```python
from build123d import *

# Parameters (mm, degrees)
SKETCH_1_R      = 6
SKETCH_1_R_2    = 5.25
EXTRUDE_2_DEPTH = 40
SKETCH_2_R      = 7.5
EXTRUDE_3_DEPTH = 3
SKETCH_3_R      = 5
EXTRUDE_4_DEPTH = 190
EXTRUDE_6_DEPTH = 1.8


with BuildPart() as part:
    # 草图1 → 凸台-拉伸2 (new body)
    with BuildSketch(Plane(origin=(0, 0, 0), x_dir=(1, 0, 0), z_dir=(0, 1, 0))):
        with Locations(Location((0, 0, 0), (0, 0, 270))):
            Circle(SKETCH_1_R)
        with Locations(Location((0, 0, 0), (0, 0, 270))):
            Circle(SKETCH_1_R_2, mode=Mode.SUBTRACT)
    extrude(amount=EXTRUDE_2_DEPTH)

    # 草图2 → 凸台-拉伸3 (add)
    with BuildSketch(Plane(origin=(0, 40, 0), x_dir=(1, 0, 0), z_dir=(0, 1, 0))):
        with Locations(Location((0, 0, 0), (0, 0, 270))):
            Circle(SKETCH_2_R)
    extrude(amount=EXTRUDE_3_DEPTH)

    # 草图3 → 凸台-拉伸4 (add)
    with BuildSketch(Plane(origin=(0, 43, 0), x_dir=(1, 0, 0), z_dir=(0, 1, 0))):
        with Locations(Location((0, 0, 0), (0, 0, 270))):
            Circle(SKETCH_3_R)
    extrude(amount=EXTRUDE_4_DEPTH)

    # 草图4 → 凸台-拉伸6 (add)
    with BuildSketch(Plane(origin=(0, 43, 0), x_dir=(1, 0, 0), z_dir=(0, 1, 0))):
        with BuildLine():
            Line((6, 2.2), (4.489988864, 2.2))
            ThreePointArc((4.489988864, 2.2), (4.870828693, 1.129171307), (5, 0))
            ThreePointArc((5, 0), (4.870828693, -1.129171307), (4.489988864, -2.2))
            Line((4.489988864, -2.2), (6, -2.2))
            Line((6, -2.2), (6, 2.2))
        make_face()
        with BuildLine():
            ThreePointArc((2.2, -4.489988864), (0, -5), (-2.2, -4.489988864))
            Line((-2.2, -4.489988864), (-2.2, -6))
            Line((-2.2, -6), (2.2, -6))
            Line((2.2, -6), (2.2, -4.489988864))
        make_face()
        with BuildLine():
            Line((-2.2, 6), (-2.2, 4.489988864))
            ThreePointArc((-2.2, 4.489988864), (0, 5), (2.2, 4.489988864))
            Line((2.2, 4.489988864), (2.2, 6))
            Line((2.2, 6), (-2.2, 6))
        make_face()
        with BuildLine():
            ThreePointArc((-4.489988864, -2.2), (-5, 0), (-4.489988864, 2.2))
            Line((-4.489988864, 2.2), (-6, 2.2))
            Line((-6, 2.2), (-6, -2.2))
            Line((-6, -2.2), (-4.489988864, -2.2))
        make_face()
    extrude(amount=EXTRUDE_6_DEPTH)


solid = part.part
```
Here's how the part is built. I have some questions about the finished solid (model axes, mm). A direction names the side the tool comes from. Coordinates: 2 decimals unless noted, no trailing zeros. Order: outer loops, then holes, each group sorted by start corner. A loop starts at its lowest first (then second) coordinate and runs counter-clockwise, first axis right, second up. Notation, with made-up numbers: (3.5, 80) - (38.5, 80) arc R28 ccw to (38.5, 99) - close; hole circle Ø2 at (80, 73.25). An arc over 180 degrees is marked (long way). One line per question, with ' | ' between items.
(1) Suppose I cut it at B-B on x = 0. List the corners of the cut face in (y, z) for me, and give its area (3 significant figures).
Report:
outline: (0, -6) - (40, -6) - (40, -7.5) - (43, -7.5) - (43, -6) - (44.8, -6) - (44.8, -5) - (233, -5) - (233, 5) - (44.8, 5) - (44.8, 6) - (43, 6) - (43, 7.5) - (40, 7.5) - (40, 6) - (0, 6) - (0, 5.25) - (40, 5.25) - (40, -5.25) - (0, -5.25) - close | area: 2,010 mm2
(2) Suppose I cut it at A-A on z = 0. List the corners of the cut face in (x, y) for me.
Report:
outline: (-7.5, 40) - (-6, 40) - (-6, 0) - (-5.25, 0) - (-5.25, 40) - (5.25, 40) - (5.25, 0) - (6, 0) - (6, 40) - (7.5, 40) - (7.5, 43) - (6, 43) - (6, 44.8) - (5, 44.8) - (5, 233) - (-5, 233) - (-5, 44.8) - (-6, 44.8) - (-6, 43) - (-7.5, 43) - close
(3) Will these pins go through, and if not, where does the flat tip stop? pin 1 (1 mm diameter, centred on x = 4, y = 186.5, fed in from +Z); pin 2 (1.5 mm diameter, centred on x = -1, y = 50.5, fed in from +Z); pin 3 (1.7 mm diameter, centred on x = -5.5, y = 44, fed in from -Z).
Report:
pin 1: stops at z = 3.57 | pin 2: stops at z = 4.99 | pin 3: stops at z = -2.2
(4) If I drill on L1, parallel to X at y = 15.5, z = 0; L2, parallel to Y at x = 1.75, z = -0.75; L3, parallel to Y at x = 7, z = -0.75, over which ranges is the centre line in solid material (lowest first)?
Report:
L1: x = -6 to -5.25, 5.25 to 6 | L2: y = 40 to 233 | L3: y = 40 to 43
(5) Suppose I cut it at C-C on y = 138. List the corners of the cut face in (x, z) for me, and give its area (3 significant figures).
Report:
outline: circle Ø10 at (0, 0) | area: 78.5 mm2
(6) For faces 1 (the flat face through (6, 40, 2)), 2 (the flat face through (0, 233, 0)), which set-ups out of +Z, -Z, +X, -X, +Y, -Y let a thin tool reach every point of the face, with its end or its side?
Report:
face 1: -Y | face 2: +Z, -Z, +X, -X, +Y
(7) If we mould it in two halves opening along X, with no side actions, what happens to faces 3 (the flat face through (0, 40, 0)), 4 (the cylindrical face through (1.5, 136.67, 4.77)), 5 (the flat face through (-4, 0, 4))? For each: pulls with the +X half, pulls with the -X half, needs draft (parallel to the pull), parting line crosses it, or undercut.
Report:
face 3: undercut | face 4: parting line crosses it | face 5: needs draft
